Input: part model. Units: mm. Frame: model coordinates. A direction names the side the tool comes from. Round coordinates to 2 decimals unless told otherwise and drop trailing zeros. Loops run counter-clockwise (first coordinate to the right, second up) from the corner with the lowest first, then second, coordinate; pieces in that order, holes last. Notation, with made-up numbers: (13.5, 31.25) -> (50.5, 31.25) arc R20 ccw to (50.5, 53.25) -> close; hole circle Ø2 at (87.5, 8). An arc over 180 degrees is marked (long way). Answer in a Markdown table with one row per item. Add a question column.
Q1. Section C-C, the plane z = 43.5. Output: boundary loops of the cut face in (x, y).
Q2. Mould query, pull axis Z, two halves, no side actions, for faces 1 (the face through (-40, 89, -63.5)), 2 (the face through (-36.5, -46.367, 60.47)), 3 (the face through (69.76, 54.39, -83.97)), 4 (the face through (-40, 124, 76.2)). Classes: pulls with the +Z half, pulls with the -Z half, needs draft (parallel to the pull), parting line crosses it, or undercut.
Q3. Pin query (flat end, axial travel): pin 1 (10 mm diameter, centred on x = -101, y = -75, fed in from +Z); pin 2 (2.5 mm diameter, centred on y = 108.5, z = -67.5, fed in from -X); pin 3 (6 mm diameter, centred on x = -98, y = -132, fed in from -Z). Return the tip coordinate at first contact, or that it passes through.
Q4. Section A-A, the plane z = 116.5. Output: boundary loops of the cut face in (x, y), and give its area (3 significant figures).
Q5. Ray query, L1, parallel to Y at x = 72.5, z = 0 (3 decimals); L2, parallel to Y at x = -23.5, z = 0; L3, parallel to Y at x = 16, z = -64. Return the intervals inside material, ascending. Write a range as from..to.
Q6. Reachability of faces 5 (the face through (-146.05, 57, -73)), 6 (the face through (-40, 72.39, 70)), 7 (the face through (-40, 112, -63.5)), 8 (the face through (-40, 129.54, 70)) from +Z, -Z, +X, -X, +Y, -Y: full face, straight path, thin tool, end or side. Return the list, or none.
Q7. Section B-B, the plane y = -107.95. Output: boundary loops of the cut face in (x, z) (3 decimals).
```python
from build123d import *

# Parameters (mm, degrees)
BOSS_EXTRUDE1_DEPTH = 165.1
BOSS_EXTRUDE2_START = 63.5
SKETCH3_R           = 88.9
SKETCH3_R_2         = 16.51
BOSS_EXTRUDE2_DEPTH = 63.5
BOSS_EXTRUDE3_START = 63.5
BOSS_EXTRUDE3_DEPTH = 209.55
SKETCH7_R           = 127
SKETCH7_R_2         = 9.525
BOSS_EXTRUDE4_DEPTH = 12.7
SKETCH8_R           = 76.2
CUT_EXTRUDE1_DEPTH  = 228.6


with BuildPart() as part:
    # Sketch2 → Boss-Extrude1 (new body)
    with BuildSketch(Plane(origin=(0, 0, 0), x_dir=(0, 0, -1), z_dir=(1, 0, 0))):
        with BuildLine():
            Line((-84.14126771, 28.695941668), (-152.4, -171.45))
            Line((-152.4, -171.45), (0, -171.45))
            Line((0, -171.45), (0, -88.9))
            ThreePointArc((0, -88.9), (-72.298959931, -51.730749007), (-84.14126771, 28.695941668))
        make_face()
        with BuildLine():
            Line((0, -88.9), (0, -171.45))
            Line((0, -171.45), (152.4, -171.45))
            Line((152.4, -171.45), (84.14126771, 28.695941668))
            ThreePointArc((84.14126771, 28.695941668), (87.702248259, 14.543921421), (88.9, 0))
            ThreePointArc((88.9, 0), (62.861792847, -62.861792847), (0, -88.9))
        make_face()
        with BuildLine():
            ThreePointArc((0, 88.9), (-51.730749007, 72.298959931), (-84.14126771, 28.695941668))
            ThreePointArc((-84.14126771, 28.695941668), (-72.298959931, -51.730749007), (0, -88.9))
            Line((0, -88.9), (0, -19.05))
            ThreePointArc((0, -19.05), (-19.05, 0), (0, 19.05))
            Line((0, 19.05), (0, 88.9))
        make_face()
        with BuildLine():
            Line((0, -19.05), (0, -88.9))
            ThreePointArc((0, -88.9), (62.861792847, -62.861792847), (88.9, 0))
            ThreePointArc((88.9, 0), (87.702248259, 14.543921421), (84.14126771, 28.695941668))
            ThreePointArc((84.14126771, 28.695941668), (51.730749007, 72.298959931), (0, 88.9))
            Line((0, 88.9), (0, 19.05))
            ThreePointArc((0, 19.05), (13.470384182, 13.470384182), (19.05, 0))
            ThreePointArc((19.05, 0), (13.470384182, -13.470384182), (0, -19.05))
        make_face()
    extrude(amount=-BOSS_EXTRUDE1_DEPTH)

    # Sketch3 → Boss-Extrude2 (add)
    with BuildSketch(Plane(origin=(0, 0, 0), x_dir=(0, 0, -1), z_dir=(1, 0, 0)).offset(BOSS_EXTRUDE2_START)):
        Circle(SKETCH3_R)
        Circle(SKETCH3_R_2, mode=Mode.SUBTRACT)
    extrude(amount=-BOSS_EXTRUDE2_DEPTH)

    # Sketch6 → Boss-Extrude3 (add)
    with BuildSketch(Plane(origin=(0, 0, 0), x_dir=(0, 0, -1), z_dir=(1, 0, 0)).offset(BOSS_EXTRUDE3_START)):
        Polygon((76.2, 152.4), (-76.2, 152.4), (-76.2, 140.97), (-63.5, 140.97), (-63.5, 129.54), (-76.2, 129.54), (-76.2, 118.11), (-63.5, 118.11), (-63.5, 106.68), (-76.2, 106.68), (-76.2, 95.25), (-63.5, 95.25), (-63.5, 83.82), (-76.2, 83.82), (-76.2, 72.39), (-63.5, 72.39), (-63.5, 61.722), (-76.2, 61.722), (-76.2, 0), (76.2, 0), (76.2, 61.722), (63.5, 61.722), (63.5, 72.39), (76.2, 72.39), (76.2, 83.82), (63.5, 83.82), (63.5, 95.25), (76.2, 95.25), (76.2, 106.68), (63.5, 106.68), (63.5, 118.11), (76.2, 118.11), (76.2, 129.54), (63.5, 129.54), (63.5, 140.97), (76.2, 140.97), align=None)
    extrude(amount=-BOSS_EXTRUDE3_DEPTH)

    # Sketch7 → Boss-Extrude4 (add)
    with BuildSketch(Plane(origin=(63.5, 0, 0), x_dir=(0, 0, -1), z_dir=(1, 0, 0))):
        with Locations(Location((0, 0, 0), (0, 0, 126.869897646))):
            Circle(SKETCH7_R)
        with Locations((0, -107.95)):
            Circle(SKETCH7_R_2, mode=Mode.SUBTRACT)
        with Locations((-93.487442339, 53.975)):
            Circle(SKETCH7_R_2, mode=Mode.SUBTRACT)
        with Locations((93.487442339, 53.975)):
            Circle(SKETCH7_R_2, mode=Mode.SUBTRACT)
    extrude(amount=BOSS_EXTRUDE4_DEPTH)

    # Sketch8 → Cut-Extrude1 (cut)
    with BuildSketch(Plane(origin=(76.2, 0, 0), x_dir=(0, 0, -1), z_dir=(1, 0, 0))):
        Circle(SKETCH8_R)
    extrude(amount=-CUT_EXTRUDE1_DEPTH, mode=Mode.SUBTRACT)


solid = part.part
```
Answer block:
| question | item | result |
|---|---|---|
| 1 | outline | (-165.1, -171.45) -> (0, -171.45) -> (0, -77.53) -> (63.5, -77.53) -> (63.5, -119.32) -> (76.2, -119.32) -> (76.2, -62.56) -> (-152.4, -62.56) -> (-152.4, 62.56) -> (76.2, 62.56) -> (76.2, 119.32) -> (63.5, 119.32) -> (63.5, 152.4) -> (-146.05, 152.4) -> (-146.05, 77.53) -> (-165.1, 77.53) -> close |
| 2 | face 1 | pulls with the -Z half |
| 2 | face 2 | undercut |
| 2 | face 3 | undercut |
| 2 | face 4 | pulls with the +Z half |
| 3 | pin 1 | z = 121.21 |
| 3 | pin 2 | x = 63.5 |
| 3 | pin 3 | z = -139.97 |
| 4 | outline | (-165.1, -171.45) -> (0, -171.45) -> (0, -66.19) -> (-165.1, -66.19) -> close; (63.5, -50.56) -> (76.2, -50.56) -> (76.2, 50.56) -> (63.5, 50.56) -> close |
| 4 | area | 18,700 mm^2 |
| 5 | L1 | -127..-117.475, -98.425..-76.2, 76.2..127 |
| 5 | L2 | -171.45..-76.2, 76.2..152.4 |
| 5 | L3 | -61.7..-41.36, 41.36..61.72, 72.39..83.82, 95.25..106.68, 118.11..129.54, 140.97..152.4 |
| 6 | face 5 | -Z, -X, +Y |
| 6 | face 6 | +Z, -X |
| 6 | face 7 | -Z, -X |
| 6 | face 8 | +Z, +X, -X |
| 7 | outline | (-165.1, -130.744) -> (0, -130.744) -> (0, 130.744) -> (-165.1, 130.744) -> close; (63.5, -66.901) -> (76.2, -66.901) -> (76.2, -9.525) -> (63.5, -9.525) -> close; (63.5, 9.525) -> (76.2, 9.525) -> (76.2, 66.901) -> (63.5, 66.901) -> close |
